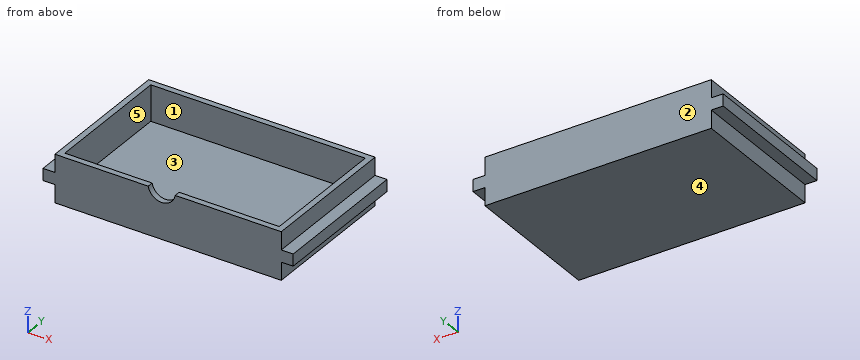
from build123d import *

# Parameters (mm, degrees)
F0_W     = 12.7
F0_H     = 12.7
F1_DEPTH = 152.4
F2_W     = 228.6
F2_H     = 139.7
F3_DEPTH = 38.1
F5_DEPTH = 6.35


with BuildPart() as f1:
    # F0 (on Front) → F1 (new body)
    with BuildSketch(Plane.XZ):
        with Locations((-154.667671, -44.050034)):
            Rectangle(F0_W, F0_H)
        Polygon((92.982329, -18.650034), (-148.317671, -18.650034), (-148.317671, -37.700034), (-148.317671, -50.400034), (-148.317671, -69.450034), (92.982329, -69.450034), (92.982329, -50.400034), (92.982329, -37.700034), align=None)
        with Locations((99.332329, -44.050034)):
            Rectangle(F0_W, F0_H)
    extrude(amount=F1_DEPTH)

    # F2 (on face) → F3 (cut)
    with BuildSketch(Plane.XY.offset(-18.650034)):
        with Locations((-27.667671, -76.2)):
            Rectangle(F2_W, F2_H)
    extrude(amount=-F3_DEPTH, mode=Mode.SUBTRACT)

    # F4 (on face) → F5 (cut)
    with BuildSketch(Plane.XZ.offset(152.4)):
        with BuildLine():
            Line((-20.082708, -18.650034), (-48.866976, -18.650034))
            ThreePointArc((-48.866976, -18.650034), (-34.474842, -30.853539), (-20.082708, -18.650034))
        make_face()
    extrude(amount=-F5_DEPTH, mode=Mode.SUBTRACT)


solid = f1.part
Model file for the job. Use its own axes, mm. Face numbers are marked on the shaded views. A direction names the side the tool comes from. Round coordinates to 2 decimals unless told otherwise and drop trailing zeros. Order: outer loops, then holes, each group sorted by start corner. A loop starts at its lowest first (then second) coordinate and runs counter-clockwise, first axis right, second up. Notation, with made-up numbers: M 13.25,70 L 55.25,70 A26 cw 55.25,95 Z; hole C 12,57.25 d6. An arc over 180 degrees is marked long. Write each question's results on one line, items separated by ' | '. Start each with the question number.
(1) Saw through at D-D, the plane z = -23.5. Give the cut face in (x, y).
(2) Saw through at C-C, the plane x = -71. Give the cut face in (y, z).
(3) Probe probe 1 along Y at (x, z) = (-15, -26); probe 2 along X at (y, z) = (-80, -33); probe 3 along X at (y, z) = (-76, -40). List the from-to ranges inside material, lowest first. Write a range as from..to.
(4) Drop flat-ended pins along their axis: pin 1 (21 mm diameter, centred on y = -88, z = -23.5, fed in from -X); pin 2 (4 mm diameter, centred on x = -156, y = -83, fed in from -Z); pin 3 (6 mm diameter, centred on x = -111, y = -110.5, fed in from +Z). Give the stop position or say it passes through.
(5) Saw through at B-B, the plane y = -101. Give the cut face in (x, z).
(6) Two-plate mould, pull along X, no slides. Class the marked faces 1, 2 and 3: pulls with the +X half, pulls with the -X half, needs draft (parallel to the pull), parting line crosses it, or undercut.
(7) Which spindle directions (+Z, -Z, +X, -X, +Y, -Y) get a long thin tool onto all of the face, cutting with end or side? Do the marked faces 4 and 5. Say none if no direction does.
(8) Saw through at A-A, the plane z = -47.5. Give the cut face in (x, y), then the cut area to 3 significant figures.
Established:
1) outline: M -148.32,-152.4 L -47.14,-152.4 L -47.14,-146.05 L -141.97,-146.05 L -141.97,-6.35 L 86.63,-6.35 L 86.63,-146.05 L -21.81,-146.05 L -21.81,-152.4 L 92.98,-152.4 L 92.98,0 L -148.32,0 Z
2) outline: M -152.4,-69.45 L 0,-69.45 L 0,-18.65 L -6.35,-18.65 L -6.35,-56.75 L -146.05,-56.75 L -146.05,-18.65 L -152.4,-18.65 Z
3) probe 1: y = -152.4..-146.05, -6.35..0 | probe 2: x = -148.32..-141.97, 86.63..92.98 | probe 3: x = -161.02..-141.97, 86.63..105.68
4) pin 1: stops at x = -148.32 | pin 2: stops at z = -50.4 | pin 3: stops at z = -56.75
5) outline: M -161.02,-50.4 L -148.32,-50.4 L -148.32,-69.45 L 92.98,-69.45 L 92.98,-50.4 L 105.68,-50.4 L 105.68,-37.7 L 92.98,-37.7 L 92.98,-18.65 L 86.63,-18.65 L 86.63,-56.75 L -141.97,-56.75 L -141.97,-18.65 L -148.32,-18.65 L -148.32,-37.7 L -161.02,-37.7 Z
6) face 1: undercut | face 2: needs draft | face 3: undercut
7) face 4: -Z, +X, -X, +Y, -Y | face 5: +Z
8) outline: M -161.02,-152.4 L 105.68,-152.4 L 105.68,0 L -161.02,0 Z; hole M -141.97,-146.05 L 86.63,-146.05 L 86.63,-6.35 L -141.97,-6.35 Z | area: 8,710 mm^2
